For this review, use the dimensioned drawing (mm, ordinates from the lowest corner) and the shaded views. A direction names the side the tool comes from. Give positions to 0.01 mm unless a question says otherwise; leave off trailing zeros. Loops run counter-clockwise (first coordinate to the right, second up) from the corner with the lowest first, then second, coordinate; pieces in that order, holes last. Notation, with made-up numbers: (26.25, -38.5) - (76.25, -38.5) arc R18 cw to (76.25, -12.5) - close; hole circle Ø2 at (77.5, -33.5). An arc over 180 degrees is marked (long way). Write each question's results on one line, items separated by ' | '.
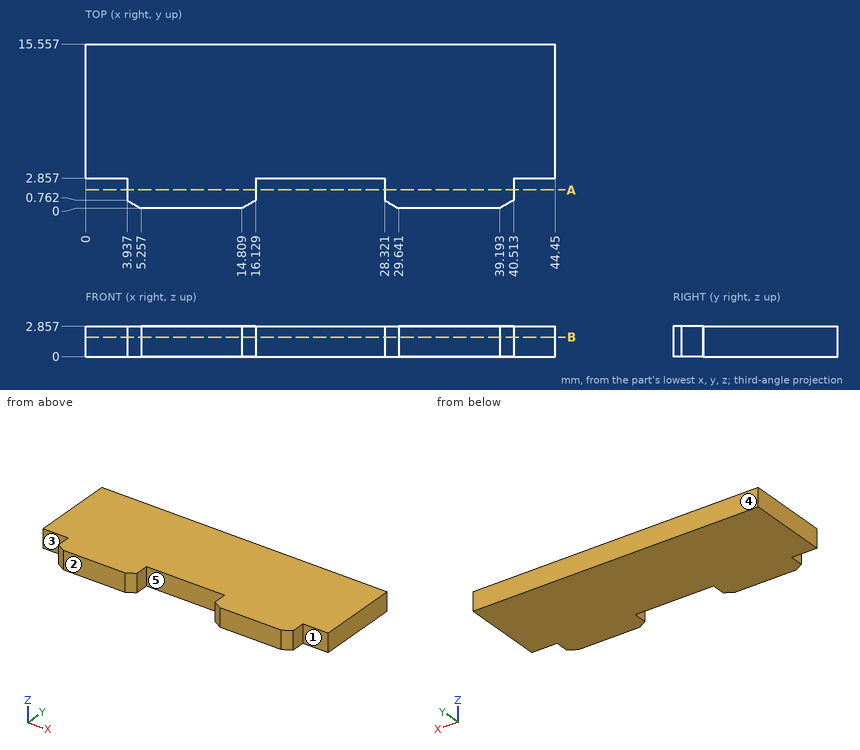
Item 1: Tool access review of the marked faces 1, 2 and 3: name each direction out of +Z, -Z, +X, -X, +Y, -Y from which nothing blocks a thin tool from reaching the whole face with its end or side.
Output values:
face 1: +Z, -Z, +X, -Y | face 2: +Z, -Z, +X, -X, -Y | face 3: +Z, -Z, -X, -Y
Item 2: We need section B-B on z = 1.85. Give the boundary of the cut face in (x, y), then the cut area to 3 significant figures.
Output values:
outline: (0, 2.86) - (3.94, 2.86) - (3.94, 0.76) - (5.26, 0) - (14.81, 0) - (16.13, 0.76) - (16.13, 2.86) - (28.32, 2.86) - (28.32, 0.76) - (29.64, 0) - (39.19, 0) - (40.51, 0.76) - (40.51, 2.86) - (44.45, 2.86) - (44.45, 15.56) - (0, 15.56) - close | area: 632 mm²
Item 3: Clearance check with flat-ended pins moving along their axes: P1, Ø0.9, axis at x = 24, z = 1.5, coming from the -Y side; P2, Ø1.7, axis at y = 1.5, z = 2, coming from the +X side; P3, Ø0.6, axis at y = 1.5, z = 2, coming from the -X side. State where each tip first meets the part, or that it passes through.
Output values:
P1: stops at y = 2.86 | P2: stops at x = 40.51 | P3: stops at x = 3.94
Item 4: We need section A-A on y = 1.75. Give the boundary of the cut face in (x, z).
Output values:
outline: (3.94, 0) - (16.13, 0) - (16.13, 2.86) - (3.94, 2.86) - close; (28.32, 0) - (40.51, 0) - (40.51, 2.86) - (28.32, 2.86) - close
Item 5: Wall thickness on probe 1 along X at (y, z) = (2.25, 1.55); probe 2 along Y at (x, z) = (23.5, 0.85); probe 3 along Y at (x, z) = (29, 2.3): over which ranges is each line inside the solid? List them lowest first.
Output values:
probe 1: x = 3.94 to 16.13, 28.32 to 40.51 | probe 2: y = 2.86 to 15.56 | probe 3: y = 0.37 to 15.56
Item 6: Draft analysis for pull direction X (two halves, no side actions). For the marked faces 4 and 5, state which applies: +X half, -X half, draft (parallel to the pull), parting line (faces both ways), or undercut.
Output values:
face 4: draft | face 5: undercut
